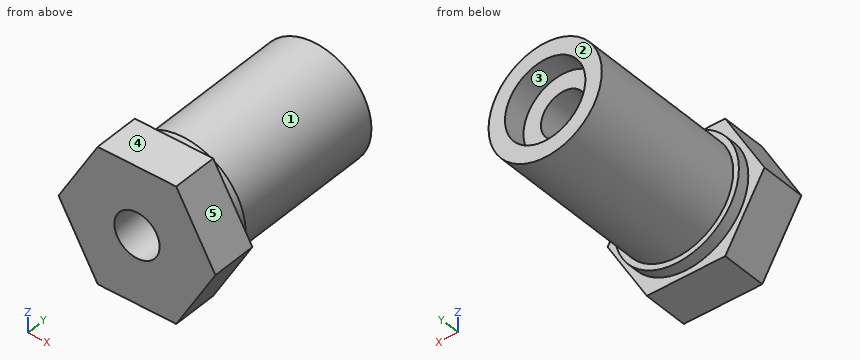
from build123d import *

# Parameters (mm, degrees)
BOSS_EXTRUDE1_DEPTH = 4
SKETCH2_R           = 5.500000049
SKETCH2_R_2         = 5.000000033
BOSS_EXTRUDE2_DEPTH = 1.016
SKETCH2_2_R         = 5.000000033
BOSS_EXTRUDE3_DEPTH = 15.24
SKETCH4_R           = 2.000000064
CUT_EXTRUDE2_DEPTH  = 20.24
SKETCH4_3_R         = 3.55
SKETCH4_3_R_2       = 2.000000064
CUT_EXTRUDE3_DEPTH  = 2


with BuildPart() as part:
    # Sketch1 → Boss-Extrude1 (new body)
    with BuildSketch(Plane(origin=(0, 0, 0), x_dir=(1, 0, 0), z_dir=(0, 1, 0))):
        Polygon((3.464101615, 6), (-3.464101615, 6), (-6.92820323, 0), (-3.464101615, -6), (3.464101615, -6), (6.92820323, 0), align=None)
    extrude(amount=BOSS_EXTRUDE1_DEPTH)

    # Sketch2 → Boss-Extrude2 (add)
    with BuildSketch(Plane(origin=(0, 4, 0), x_dir=(1, 0, 0), z_dir=(0, 1, 0))):
        Circle(SKETCH2_R)
        Circle(SKETCH2_R_2, mode=Mode.SUBTRACT)
    extrude(amount=BOSS_EXTRUDE2_DEPTH)

    # Sketch2<2> → Boss-Extrude3 (add)
    with BuildSketch(Plane(origin=(0, 4, 0), x_dir=(1, 0, 0), z_dir=(0, 1, 0))):
        Circle(SKETCH2_2_R)
    extrude(amount=BOSS_EXTRUDE3_DEPTH)

    # Sketch4 → Cut-Extrude2 (cut, through all)
    with BuildSketch(Plane(origin=(0, 19.24, 0), x_dir=(1, 0, 0), z_dir=(0, 1, 0))):
        Circle(SKETCH4_R)
    extrude(amount=-CUT_EXTRUDE2_DEPTH, mode=Mode.SUBTRACT)

    # Sketch4<3> → Cut-Extrude3 (cut)
    with BuildSketch(Plane(origin=(0, 19.24, 0), x_dir=(1, 0, 0), z_dir=(0, 1, 0))):
        Circle(SKETCH4_3_R)
        Circle(SKETCH4_3_R_2, mode=Mode.SUBTRACT)
    extrude(amount=-CUT_EXTRUDE3_DEPTH, mode=Mode.SUBTRACT)


solid = part.part
Geometry: final body of the model. Coordinates: model frame, mm. Face numbers are marked on the shaded views. A direction names the side the tool comes from. Round coordinates to 2 decimals unless told otherwise and drop trailing zeros. Write each loop counter-clockwise with the first axis right and the second up, starting at its lowest first coordinate (ties: lowest second). Pieces come first, ordered by that corner, then holes. Notation, with made-up numbers: M 75.25,-4 L 124.25,-4 A13 ccw 124.25,7 Z; hole C 48,55 d5. An arc over 180 degrees is marked long. Write item = value, one per line.
Item 1: Section query B-B on z = 1. Return loops of the section in (x, y).
Findings:
outline = M -6.35,0 L -1.73,0 L -1.73,17.24 L -3.41,17.24 L -3.41,19.24 L -4.9,19.24 L -4.9,5.02 L -5.41,5.02 L -5.41,4 L -6.35,4 Z; M 1.73,0 L 6.35,0 L 6.35,4 L 5.41,4 L 5.41,5.02 L 4.9,5.02 L 4.9,19.24 L 3.41,19.24 L 3.41,17.24 L 1.73,17.24 Z
Item 2: Access query for the marked faces 1 and 2. Directions: +Z, -Z, +X, -X, +Y, -Y. A direction counts if a zero-diameter tool reaches every point of the face in a straight line with its end or side. Return the directions, or none.
Findings:
face_1 = +Y
face_2 = +Z, -Z, +X, -X, +Y
Item 3: Material intervals for line 1 along Z through (x, y) = (0, 9.5); line 2 along Z through (x, y) = (0, 18.55), sorted ascending. Write a range as [from, to].
Findings:
line_1 = [-5, -2], [2, 5]
line_2 = [-5, -3.55], [3.55, 5]
Item 4: Pull-direction query (X, two-part tool) for the marked faces 3, 4 and 5; classes: pulls with the +X half, pulls with the -X half, needs draft (parallel to the pull), parting line crosses it, or undercut.
Findings:
face_3 = undercut
face_4 = needs draft
face_5 = pulls with the +X half
Item 5: Section query C-C on z = -2.5. Return loops of the section in (x, y).
Findings:
outline = M -5.48,0 L 5.48,0 L 5.48,4 L 4.9,4 L 4.9,5.02 L 4.33,5.02 L 4.33,19.24 L 2.52,19.24 L 2.52,17.24 L -2.52,17.24 L -2.52,19.24 L -4.33,19.24 L -4.33,5.02 L -4.9,5.02 L -4.9,4 L -5.48,4 Z
Item 6: Pin query (flat end, axial travel): P1, Ø1, axis at y = 9, z = 3.5, coming from the +X side; P2, Ø3.5, axis at x = 0.5, z = -1.5, coming from the +Y side; P3, Ø1, axis at x = -4.5, y = 4, coming from the +Z side. Return the tip coordinate at first contact, or that it passes through.
Findings:
P1 = 4
P2 = 17.24
P3 = 5.07
Item 7: Section query A-A on x = 0. Return loops of the section in (y, z).
Findings:
outline = M 0,-6 L 4,-6 L 4,-5.5 L 5.02,-5.5 L 5.02,-5 L 19.24,-5 L 19.24,-3.55 L 17.24,-3.55 L 17.24,-2 L 0,-2 Z; M 0,2 L 17.24,2 L 17.24,3.55 L 19.24,3.55 L 19.24,5 L 5.02,5 L 5.02,5.5 L 4,5.5 L 4,6 L 0,6 Z
Item 8: Section query D-D on x = -2.75. Return loops of the section in (y, z) (3 decimals).
Findings:
outline = M 0,-6 L 4,-6 L 4,-4.763 L 5.016,-4.763 L 5.016,-4.176 L 19.24,-4.176 L 19.24,-2.245 L 17.24,-2.245 L 17.24,2.245 L 19.24,2.245 L 19.24,4.176 L 5.016,4.176 L 5.016,4.763 L 4,4.763 L 4,6 L 0,6 Z
